Solid Edge part; units mm, degrees
sketch "Sketch1" plane through (0, 0, 0) normal (0, 0, 1) x (1, 0, 0)
  circle A0 centre (0, 0) radius 1.5
extrude "Protrusion1" add sketch "Sketch1" along normal blind 5
sketch "Sketch2" plane through (0, 0, 5) normal (0, 0, 1) x (1, 0, 0)
  line L0 (2.25, 1.299) -> (0, 2.5981)
  line L1 (0, 2.5981) -> (-2.25, 1.299)
  line L2 (-2.25, 1.299) -> (-2.25, -1.299)
  line L3 (-2.25, -1.299) -> (0, -2.5981)
  line L4 (0, -2.5981) -> (2.25, -1.299)
  line L5 (2.25, -1.299) -> (2.25, 1.299)
extrude "ExtrudedProtrusion_2" add sketch "Sketch2" along normal blind 44
sketch "Sketch3" plane through (0, 0, 49) normal (0, 0, 1) x (0, 1, 0)
  circle A0 centre (0, 0) radius 1.5
extrude "ExtrudedCutout_1" cut sketch "Sketch3" against normal blind 10
fillet "Round_1" radius 0.2 20 edges at (2.25, -1.299, 27) (2.25, 1.299, 27) (2.25, 0, 49) (1.125, 1.9486, 49) (0, -1.5, 49) (0, 2.5981, 27) (1.125, 1.9486, 5) (2.25, 0, 5) (1.125, -1.9486, 5) (0, -2.5981, 27) (1.125, -1.9486, 49) (-1.125, -1.9486, 49) (-1.125, -1.9486, 5) (-2.25, -1.299, 27) (-2.25, 0, 49) (-1.125, 1.9486, 49) (-2.25, 1.299, 27) (-2.25, 0, 5) (-1.125, 1.9486, 5) (-1.5, 0, 0)
properties material "Brass, yellow brass"
The model under review builds one solid part; all positions refer to its coordinate system, in mm. A direction names the side the tool comes from. Round coordinates to 2 decimals unless told otherwise and drop trailing zeros. Order: outer loops, then holes, each group sorted by start corner. A loop starts at its lowest first (then second) coordinate and runs counter-clockwise, first axis right, second up. Notation, with made-up numbers: (73.25, -7) -> (109.25, -7) arc R30 ccw to (109.25, 25) -> close; hole circle Ø2 at (5, 13). An arc over 180 degrees is marked (long way). One line per item, written item: value. Start each with the question number.
Q1. Machinability: for faces 4 (the face through (-0.07, -1.5, 43.97)), 5 (the face through (0, -2, 49)), 6 (the face through (0, -2, 5)), which of the approach directions +Z, -Z, +X, -X, +Y, -Y give a long, thin tool a straight path to every point of the face, cutting with its end or side? Answer none if there is none.
Q2. Take a section at B-B (y = 0). Write out the cut boundary in (x, z).
Q3. Take a section at A-A (z = 40.5). Write out the cut boundary in (x, y), and give its area (3 significant figures).
Q4. Take a section at C-C (z = 26). Write out the cut boundary in (x, y).
Q5. Mouldability with a two-part tool opening along Y and no side actions: class faces 1 (the face through (0, 0, 0)), 2 (the face through (0, 0, 39)), 3 (the face through (-1.11, 1.89, 5.06)) as released by +Y, released by -Y, zero draft, split by the parting line, or undercut.
Q6. Wall thickness on line 1 (Y direction, x = 0, z = 42.5); line 2 (X direction, y = 0, z = 44.75); line 3 (Z direction, x = -0.5, y = -1.7): over which ranges is each line inside the solid? List them lowest first.
Reported:
1. face 4: +Z
1. face 5: +Z, +X, -X, +Y, -Y
1. face 6: -Z
2. outline: (-2.25, 5.2) arc R0.2 ccw to (-2.05, 5) -> (-1.5, 5) -> (-1.5, 0.2) arc R0.2 ccw to (-1.3, 0) -> (1.3, 0) arc R0.2 ccw to (1.5, 0.2) -> (1.5, 5) -> (2.05, 5) arc R0.2 ccw to (2.25, 5.2) -> (2.25, 48.8) arc R0.2 ccw to (2.05, 49) -> (1.7, 49) arc R0.2 ccw to (1.5, 48.8) -> (1.5, 39) -> (-1.5, 39) -> (-1.5, 48.8) arc R0.2 ccw to (-1.7, 49) -> (-2.05, 49) arc R0.2 ccw to (-2.25, 48.8) -> close
3. outline: (-2.25, -1.18) arc R0.2 ccw to (-2.15, -1.36) -> (-0.1, -2.54) arc R0.2 ccw to (0.1, -2.54) -> (2.15, -1.36) arc R0.2 ccw to (2.25, -1.18) -> (2.25, 1.18) arc R0.2 ccw to (2.15, 1.36) -> (0.1, 2.54) arc R0.2 ccw to (-0.1, 2.54) -> (-2.15, 1.36) arc R0.2 ccw to (-2.25, 1.18) -> close; hole circle Ø3 at (0, 0)
3. area: 10.5 mm2
4. outline: (-2.25, -1.18) arc R0.2 ccw to (-2.15, -1.36) -> (-0.1, -2.54) arc R0.2 ccw to (0.1, -2.54) -> (2.15, -1.36) arc R0.2 ccw to (2.25, -1.18) -> (2.25, 1.18) arc R0.2 ccw to (2.15, 1.36) -> (0.1, 2.54) arc R0.2 ccw to (-0.1, 2.54) -> (-2.15, 1.36) arc R0.2 ccw to (-2.25, 1.18) -> close
5. face 1: zero draft
5. face 2: undercut
5. face 3: released by +Y
6. line 1: y = -2.57 to -1.5, 1.5 to 2.57
6. line 2: x = -2.25 to -1.5, 1.5 to 2.25
6. line 3: z = 5 to 49
